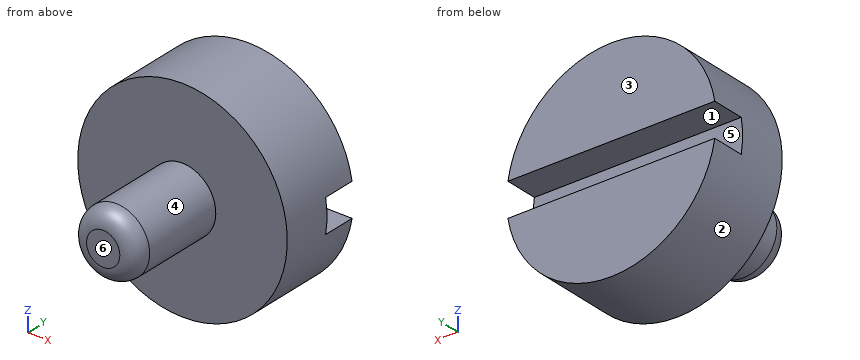
```python
from build123d import *

# Parameters (mm, degrees)
SKETCH1_R           = 2.54
BOSS_EXTRUDE1_DEPTH = 7.62
SKETCH2_R           = 8.001
BOSS_EXTRUDE2_DEPTH = 6.35
FILLET1_R           = 1.27
SKETCH3_W           = 2.54
SKETCH3_H           = 2.54
CUT_EXTRUDE1_DEPTH  = 63.5


with BuildPart() as part:
    # Sketch1 → Boss-Extrude1 (new body)
    with BuildSketch(Plane(origin=(0, 0, 0), x_dir=(1, 0, 0), z_dir=(0, 1, 0))):
        with Locations(Location((0, 0, 0), (0, 0, 90))):
            Circle(SKETCH1_R)
    extrude(amount=BOSS_EXTRUDE1_DEPTH)

    # Sketch2 → Boss-Extrude2 (add)
    with BuildSketch(Plane(origin=(0, 7.62, 0), x_dir=(1, 0, 0), z_dir=(0, 1, 0))):
        with Locations(Location((0, 0, 0), (0, 0, 270))):
            Circle(SKETCH2_R)
    extrude(amount=BOSS_EXTRUDE2_DEPTH)

    # Fillet1
    fillet1_edges = [part.edges().sort_by_distance(p)[0] for p in [
        (0, 0, 2.54),
    ]]
    fillet(fillet1_edges, radius=FILLET1_R)

    # Sketch3 → Cut-Extrude1 (cut, symmetric)
    with BuildSketch(Plane(origin=(0, 0, 0), x_dir=(0, 0, -1), z_dir=(1, 0, 0))):
        with Locations((0, 12.7)):
            Rectangle(SKETCH3_W, SKETCH3_H)
    extrude(amount=CUT_EXTRUDE1_DEPTH, both=True, mode=Mode.SUBTRACT)


solid = part.part
```
Geometry check sheet. Reference: the model listing, model coordinates, mm. Face numbers are marked on the shaded views. A direction names the side the tool comes from. Coordinates: 2 decimals unless noted, no trailing zeros. Order: outer loops, then holes, each group sorted by start corner. A loop starts at its lowest first (then second) coordinate and runs counter-clockwise, first axis right, second up. Notation, with made-up numbers: (63.5, 88.25) - (71.5, 88.25) arc R29 ccw to (71.5, 125.25) - close; hole circle Ø9 at (60.5, 66). An arc over 180 degrees is marked (long way). Answer in a Markdown table with one row per item. Add a question column.
1. Section check D-D (x = -5). Enter the section's corners in (y, z), plus the area to 3 significant figures.
2. Section check A-A (x = 4). Enter the section's corners in (y, z).
3. Gauge pin test, flat ends, axial feed: pin 1 Ø1.5 at (x, y) = (4, 6.5) entering from -Z; pin 2 Ø1 at (x, y) = (4.5, 12) entering from +Z; pin 3 Ø6 at (y, z) = (3, 3) entering from +X; pin 4 Ø5 at (x, z) = (-3, -2.5) entering from -Y. Record the tip position at first contact, or that the pin passes through.
4. Section check C-C (z = -6). Enter the section's corners in (x, y).
5. Draft check along Z on the marked faces 1, 2 and 3. Enter one of: +Z half, -Z half, draft (parallel to the pull), parting line (faces both ways), or undercut.
6. Access from +Z, -Z, +X, -X, +Y, -Y to the whole of each face (thin tool, end or side, straight path). Record for the marked faces 4, 5 and 6.
7. Section check B-B (y = 4). Enter the section's corners in (x, z).
8. Material ranges on L1, parallel to Y at x = -1, z = 6.25; L2, parallel to X at y = 6, z = 0; L3, parallel to Y at x = 3.25, z = -0.5, recorded low to high. Write a range as [from, to].
Data:
| question | item | result |
|---|---|---|
| 1 | outline | (7.62, -6.25) - (13.97, -6.25) - (13.97, -1.27) - (11.43, -1.27) - (11.43, 1.27) - (13.97, 1.27) - (13.97, 6.25) - (7.62, 6.25) - close |
| 1 | area | 72.9 mm² |
| 2 | outline | (7.62, -6.93) - (13.97, -6.93) - (13.97, -1.27) - (11.43, -1.27) - (11.43, 1.27) - (13.97, 1.27) - (13.97, 6.93) - (7.62, 6.93) - close |
| 3 | pin 1 | passes through |
| 3 | pin 2 | stops at z = 6.93 |
| 3 | pin 3 | stops at x = 2.54 |
| 3 | pin 4 | stops at y = 0.01 |
| 4 | outline | (-5.29, 7.62) - (5.29, 7.62) - (5.29, 13.97) - (-5.29, 13.97) - close |
| 5 | face 1 | undercut |
| 5 | face 2 | parting line |
| 5 | face 3 | draft |
| 6 | face 4 | -Y |
| 6 | face 5 | +X, -X, +Y |
| 6 | face 6 | +Z, -Z, +X, -X, -Y |
| 7 | outline | circle Ø5.08 at (0, 0) |
| 8 | L1 | y = [7.62, 13.97] |
| 8 | L2 | x = [-2.54, 2.54] |
| 8 | L3 | y = [7.62, 11.43] |
